Check sheet for the modelled part. Datum: model origin and axes. Units: mm. Coordinates: 2 decimals unless noted, no trailing zeros. Loops run counter-clockwise (first coordinate to the right, second up) from the corner with the lowest first, then second, coordinate; pieces in that order, holes last. Notation, with made-up numbers: (15, 39.5) -> (50, 39.5) arc R20 ccw to (50, 44.5) -> close; hole circle Ø2 at (7, 17.5). An arc over 180 degrees is marked (long way). Use CSV: the item, a comma, the result in double quotes.
```python
from build123d import *

# Parameters (mm, degrees)
SKETCH1_R           = 55
BOSS_EXTRUDE1_DEPTH = 1
FILLET2_R           = 0.2
SKETCH4_R           = 5.25
CUT_EXTRUDE2_DEPTH  = 78.78817405
SKETCH5_R           = 1.3
CUT_EXTRUDE3_DEPTH  = 1


with BuildPart() as part:
    # Sketch1 → Boss-Extrude1 (new body)
    with BuildSketch(Plane(origin=(0, 0, 0), x_dir=(1, 0, 0), z_dir=(0, 1, 0))):
        with Locations(Location((0, 0, 0), (0, 0, 270))):
            Circle(SKETCH1_R)
    extrude(amount=BOSS_EXTRUDE1_DEPTH)

    # Fillet2
    fillet2_edges = [part.edges().sort_by_distance(p)[0] for p in [
        (0, 0, -55),
        (0, 1, -55),
    ]]
    fillet(fillet2_edges, radius=FILLET2_R)

    # Sketch4 → Cut-Extrude2 (cut, through all)
    with BuildSketch(Plane(origin=(0, 1, 0), x_dir=(1, 0, 0), z_dir=(0, 1, 0))):
        with Locations(Location((0, 0, 0), (0, 0, 270))):
            Circle(SKETCH4_R)
    extrude(amount=-CUT_EXTRUDE2_DEPTH, mode=Mode.SUBTRACT)

    # Sketch5 → Cut-Extrude3 (cut)
    with BuildSketch(Plane(origin=(0, 1, 0), x_dir=(1, 0, 0), z_dir=(0, 1, 0))):
        with Locations(Location((-10.900916731, 0, 0), (0, 0, 270))):
            Circle(SKETCH5_R)
        with Locations(Location((0, 11.05, 0), (0, 0, 270))):
            Circle(SKETCH5_R)
        with Locations(Location((11.05, 0, 0), (0, 0, 270))):
            Circle(SKETCH5_R)
        with Locations(Location((0, -11.05, 0), (0, 0, 270))):
            Circle(SKETCH5_R)
    extrude(amount=-CUT_EXTRUDE3_DEPTH, mode=Mode.SUBTRACT)


solid = part.part
```
1) Thickness scan on line 1 along X through (y, z) = (0.25, 0); line 2 along Z through (x, y) = (1, 0.35); line 3 along X through (y, z) = (0.2, 2.5). Record the ranges inside material, lowest first. Write a range as from..to.
Answer below:
line 1,"x = -55..-12.2, -9.6..-5.25, 5.25..9.75, 12.35..55"
line 2,"z = -54.99..-11.88, -10.22..-5.15, 5.15..10.22, 11.88..54.99"
line 3,"x = -54.94..-4.62, 4.62..54.94"
2) Cross-section at A-A on z = 0. Record the boundary of the cut face in (x, y), and give its area (3 significant figures).
Answer below:
outline,"(-55, 0.2) arc R0.2 ccw to (-54.8, 0) -> (-12.2, 0) -> (-12.2, 1) -> (-54.8, 1) arc R0.2 ccw to (-55, 0.8) -> close; (-9.6, 0) -> (-5.25, 0) -> (-5.25, 1) -> (-9.6, 1) -> close; (5.25, 0) -> (9.75, 0) -> (9.75, 1) -> (5.25, 1) -> close; (12.35, 0) -> (54.8, 0) arc R0.2 ccw to (55, 0.2) -> (55, 0.8) arc R0.2 ccw to (54.8, 1) -> (12.35, 1) -> close"
area,"94.3 mm²"
3) Draft check along X on faces 1 (the cylindrical face through (-48.794, 0.496, 25.379)), 2 (the cylindrical face through (0.06, 0.51, -12.35)), 3 (the flat face through (13, 1, -1)), 4 (the cylindrical face through (1.6, 0.5, 5)). Enter one of: released by +X, released by -X, zero draft, split by the parting line, or undercut.
Answer below:
face 1,"split by the parting line"
face 2,"undercut"
face 3,"zero draft"
face 4,"undercut"
4) Cross-section at B-B on y = 0.45. Record the boundary of the cut face in (x, z).
Answer below:
outline,"circle Ø110 at (0, 0); hole circle Ø2.6 at (-10.9, 0); hole circle Ø10.5 at (0, 0); hole circle Ø2.6 at (0, -11.05); hole circle Ø2.6 at (0, 11.05); hole circle Ø2.6 at (11.05, 0)"
5) Go/stop test with a flat-tipped pin: pin 1 Ø2.5 at (x, z) = (11.05, 0) entering from +Y. Record where the tip stops, or that it passes through.
Answer below:
pin 1,"passes through"
